Can you work these out from the model? Positions are in its coordinate system, mm. Face numbers are marked on the shaded views. Give positions to 0.01 mm unless a question says otherwise; leave off trailing zeros. Order: outer loops, then holes, each group sorted by start corner. A loop starts at its lowest first (then second) coordinate and runs counter-clockwise, first axis right, second up. Notation, with made-up numbers: M -19,28 L -6,28 A24 ccw -6,63 Z; hole C 4,-34.75 d3. An arc over 180 degrees is marked long. Use one line per item in the form item = value. Start each with the question number.
1. I want a section at C-C, the plane z = -3.5. List the corners of the cut face in (x, y) for me, and give its area (3 significant figures).
2. I want a section at A-A, the plane x = 0. List the corners of the cut face in (y, z) for me.
3. We'd pull the mould along Y, two halves only. Please class the marked faces 1, 2, 3 and 4: +Y half, -Y half, draft (parallel to the pull), parting line (faces both ways), or undercut.
4. I need wall thicknesses on L1, parallel to Y at x = 0, z = -8; L2, parallel to X at y = -3, z = -12. Which ranges of each line are inside material? Lowest first, please.
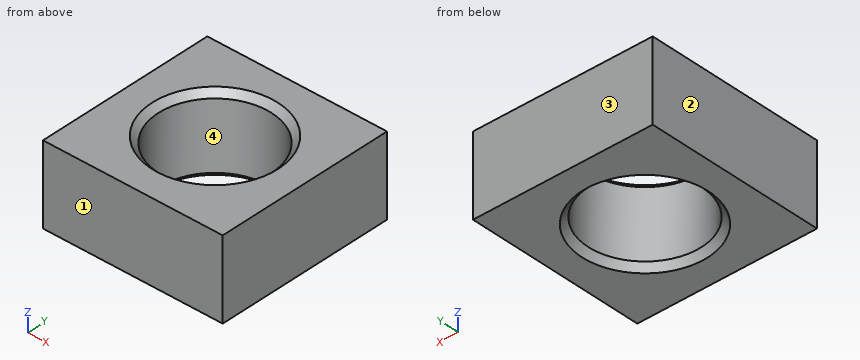
```python
from build123d import *

# Parameters (mm, degrees)
SKETCH_W            = 28.575
SKETCH_H            = 28.575
BOSS_EXTRUDE1_DEPTH = 12.7


with BuildPart() as part:
    # Sketch → Boss-Extrude1 (new body)
    with BuildSketch(Plane.XY):
        Rectangle(SKETCH_W, SKETCH_H)
    extrude(amount=-BOSS_EXTRUDE1_DEPTH)

    # Sketch1 → M20x2.0 Tapped Hole1 (revolve, cut)
    with BuildSketch(Plane(origin=(0, 0, 0), x_dir=(0, -1, 0), z_dir=(1, 0, 0))):
        Polygon((0, 0), (0, 12.7), (10, 12.7), (9, 11.7), (9, 1), (10, 0), align=None)
    revolve(axis=Axis((0, 0, 6.35), (0, 0, -1)), mode=Mode.SUBTRACT)


solid = part.part
```
Check result:
q1.outline = M -14.29,-14.29 L 14.29,-14.29 L 14.29,14.29 L -14.29,14.29 Z; hole C 0,0 d18
q1.area = 562 mm2
q2.outline = M -14.29,-12.7 L -10,-12.7 L -9,-11.7 L -9,-1 L -10,0 L -14.29,0 Z; M 9,-11.7 L 10,-12.7 L 14.29,-12.7 L 14.29,0 L 10,0 L 9,-1 Z
q3.face_1 = -Y half
q3.face_2 = draft
q3.face_3 = +Y half
q3.face_4 = undercut
q4.L1 = -14.29 to -9, 9 to 14.29
q4.L2 = -14.29 to -8.8, 8.8 to 14.29
